Autodesk Inventor part; units mm, degrees
ref_plane "Work Plane1" through (-106.5, -37, 0) normal (1, 0, 0) x (0, 1, 0)
ref_plane "Work Plane2" through (-183, -37, 0) normal (1, 0, 0) x (0, 1, 0)
ref_plane "Work Plane3" through (-106.5, -37, -17.5) normal (0, -1, 0) x (1, 0, 0)
sketch "Sketch1" plane through (0, 0, 0) normal (0, 0, 1) x (1, 0, 0)
  line L0 (-183, -19.5) -> (-106.5, -19.5)
  line L1 (-106.5, -19.5) -> (-106.5, -54.5)
  line L2 (-106.5, -54.5) -> (-183, -54.5)
  line L3 (-183, -54.5) -> (-183, -19.5)
  line L4 (-194, -37) -> (-96, -37) construction
  line L5 (-183, -22) -> (-157.5, -22)
  line L6 (-157.5, -22) -> (-157.5, -37)
  line L7 (-157.5, -24.5) -> (-116.5, -24.5)
  line L8 (-116.5, -37) -> (-116.5, -22)
  line L9 (-116.5, -22) -> (-106.5, -22)
  line L10 (-183, -52) -> (-157.5, -52) construction
  line L11 (-157.5, -52) -> (-157.5, -37) construction
  line L12 (-157.5, -49.5) -> (-116.5, -49.5) construction
  line L13 (-116.5, -37) -> (-116.5, -52) construction
  line L14 (-116.5, -52) -> (-106.5, -52) construction
  line L15 (-183, -37) -> (-106.5, -37)
  point P0 (0, 0)
  dimension "d0" = 76.5
  dimension "d1" = 35
  dimension "d2" = 30
  dimension "d3" = 25.5
  dimension "d4" = 10
  dimension "d5" = 25
  dimension "d6" = 30
sketch "Sketch3" plane through (0, 0, 0) normal (1, 0, 0) x (0, 1, 0)
  point P0 (0, 0)
ref_plane "Work Plane1" through (-106.5, -37, 0) normal (1, 0, 0) x (0, 1, 0)
sketch "Sketch4" plane through (-106.5, -37, 0) normal (1, 0, 0) x (0, 1, 0)
  point P0 (37, 0)
sketch "Sketch5" plane through (-106.5, -37, 0) normal (1, 0, 0) x (0, 1, 0)
  line L0 (-17.5, 17.5) -> (17.5, 17.5)
  line L1 (17.5, 17.5) -> (17.5, -17.5)
  line L2 (17.5, -17.5) -> (-17.5, -17.5)
  line L3 (-17.5, -17.5) -> (-17.5, 17.5)
  line L4 (-17.5, 17.5) -> (17.5, -17.5) construction
  line L5 (17.5, 17.5) -> (-17.5, -17.5) construction
  point P0 (37, 0)
  point P1 (0, 0)
  dimension "d10" = 35
  dimension "d11" = 35
ref_plane "Work Plane2" through (-183, -37, 0) normal (1, 0, 0) x (0, 1, 0)
extrude "Extrusion1" add sketch "Sketch5" against normal up to surface (76.5 mm away)
revolve "Revolution2" cut sketch "Sketch1" angle 360 about axis through (-194, -37, 0) along (1, 0, 0) contours L5 L6 L15 L3 | L1 L15 L8 L9 | L6 L7 L8 L15
sketch "Sketch7" plane through (-106.5, -37, 0) normal (1, 0, 0) x (0, 0, -1)
  circle A0 centre (0, 0) radius 19.09
  line L0 (-17.5, -17.5) -> (17.5, -17.5)
  line L1 (-17.5, 17.5) -> (-17.5, -17.5)
  line L2 (17.5, -17.5) -> (-17.5, 17.5) construction
  circle A1 centre (13.4987, -13.4987) radius 1.5
  circle A2 centre (13.4987, 13.4987) radius 1.5
  circle A3 centre (-13.4987, 13.4987) radius 1.5
  circle A4 centre (-13.4987, -13.4987) radius 1.5
  point P0 (0, 37)
  dimension "d21" = 38.18
  dimension "d22" = 3
  dimension "d25" = 360
hole "Hole1" at (-106.5, -23.5013, -13.4987) at (-106.5, -23.5013, 13.4987) at (-106.5, -50.4987, 13.4987) at (-106.5, -50.4987, -13.4987) direction (-1, 0, 0) diameter 2.8 depth 7 tip angle 118 counterbore diameter 3 counterbore depth 5
sketch "Sketch8" plane through (-183, -54.5, -17.5) normal (-1, 0, 0) x (0, 0, 1)
  line L0 (17.5, -7) -> (17.5, 46)
  circle A0 centre (2.5, 30) radius 1.25
  line L1 (0, 35) -> (0, 0)
  line L2 (35, 35) -> (0, 35)
  circle A1 centre (32.5, 30) radius 1.25
  circle A2 centre (17.5, 17.5) radius 15
  circle A3 centre (17.5, 17.5) radius 15
  line L3 (5.3, 6.5) -> (5.3, 35)
  line L4 (0, 35) -> (35, 35)
  arc A4 (5.3, 6.5) -> (6.3, 5.5) centre (6.3, 6.5) ccw
  line L5 (17.5, 5.5) -> (6.3, 5.5)
  line L6 (29.7, 6.5) -> (29.7, 35)
  arc A5 (28.7, 5.5) -> (29.7, 6.5) centre (28.7, 6.5) ccw
  line L7 (17.5, 5.5) -> (28.7, 5.5)
  point P0 (17.5, 54.5)
  point P1 (17.5, 5.5)
  point P2 (5.3, 35)
  dimension "d34" = 2.5
  dimension "d35" = 2.5
  dimension "d36" = 5
  dimension "d38" = 1
  dimension "d39" = 29.5
  dimension "d40" = 24.4
extrude "Extrusion2" cut sketch "Sketch8" against normal blind 2.75 contours L5 A2 L3 L0 | L0 A2 L6 L7 | L5 A4 L3 A2 | A2 L6 A5 L7 | A2 L3 L2 L0 | L0 L2 L6 A2
hole "Hole2" at (-183, -24.5, -15) at (-183, -24.5, 15) direction (1, 0, 0) diameter 2 depth 5 tip angle 118 counterbore diameter 2.5 counterbore depth 4
ref_plane "Work Plane3" through (-106.5, -37, -17.5) normal (0, -1, 0) x (1, 0, 0)
sketch "Sketch9" plane through (-106.5, -37, -17.5) normal (0, -1, 0) x (1, 0, 0)
  point P0 (106.5, 17.5)
sketch "Sketch11" plane through (-106.5, -19.5, 17.5) normal (0, 1, 0) x (1, 0, 0)
  line L0 (-73.75, 5.3) -> (-76.5, 5.3)
  line L1 (-76.5, 0) -> (-76.5, 5.3)
  line L2 (0, 0) -> (-76.5, 0)
  line L3 (0, 35) -> (0, 0)
  line L4 (0, 35) -> (-76.5, 35)
  line L5 (-76.5, 29.7) -> (-76.5, 35)
  line L6 (-76.5, 29.7) -> (-73.75, 29.7)
  line L7 (-73.75, 29.7) -> (-73.75, 5.3)
  line L8 (28.2317, 17.5) -> (-103.7683, 17.5) construction
  circle A0 centre (-30, 17.5) radius 1.5
  circle A1 centre (-50, 17.5) radius 2.5
  point P0 (106.5, 17.5)
  point P1 (0, 17.5)
  dimension "d54" = 3
  dimension "d55" = 5
  dimension "d56" = 30
  dimension "d57" = 50
extrude "Extrusion3" cut sketch "Sketch11" against normal up to surface (35 mm away) contours A0
extrude "Extrusion4" cut sketch "Sketch11" against normal up to surface contours A1
sketch "Sketch12" plane through (-106.5, -54.5, -17.5) normal (0, 0, -1) x (-1, 0, 0)
  line L0 (76.5, 35) -> (76.5, 0)
  line L1 (0, 35) -> (76.5, 35)
  line L2 (0, 0) -> (0, 35)
  line L3 (0, 0) -> (76.5, 0)
  line L4 (-16, 17.5) -> (90, 17.5)
  circle A0 centre (15, 5) radius 1.5
  circle A1 centre (45, 5) radius 1.5
  circle A2 centre (15, 30) radius 1.5
  circle A3 centre (45, 30) radius 1.5
  point P0 (-106.5, 54.5)
  point P1 (0, 17.5)
  dimension "d62" = 3
  dimension "d63" = 15
  dimension "d64" = 5
  dimension "d67" = 30
hole "Hole3" at (-121.5, -24.5, -17.5) at (-151.5, -24.5, -17.5) at (-151.5, -49.5, -17.5) at (-121.5, -49.5, -17.5) direction (0, 0, 1) diameter 2.8 depth 7 tip angle 118 counterbore diameter 3 counterbore depth 5
ref_plane "Work Plane4" through (-106.5, -54.5, 0) normal (0, 0, -1) x (-1, 0, 0)
mirror "Mirror2" about plane through (-106.5, -54.5, 0) normal (0, 0, -1) of "Hole3"
chamfer "Chamfer3" distance 0.5 angle 45 4 edges at (-151.5, -51, -17.5) (-151.5, -26, -17.5) (-121.5, -51, -17.5) (-121.5, -26, -17.5) measured on face at (-172.9115, -40.8826, -17.5)
chamfer "Chamfer4" distance 0.5 angle 45 4 edges at (-151.5, -26, 17.5) (-151.5, -51, 17.5) (-121.5, -26, 17.5) (-121.5, -51, 17.5) measured on face at (-172.9115, -33.1174, 17.5)
chamfer "Chamfer5" distance 0.5 angle 45 4 edges at (-106.5, -50.4987, -11.9987) (-106.5, -23.5013, -11.9987) (-106.5, -50.4987, 14.9987) (-106.5, -23.5013, 14.9987) measured on face at (-106.5, -37.6027, 16.6302)
chamfer "Chamfer6" distance 0.2 angle 45 1 edges at (-159, -19.5, 0) measured on face at (-148.5662, -19.5, -12.4939)
equation "\"d27\" = m3"
equation "\"d72\" = m3"
equation "\"m3\" = 2.8"
equation "\"m4\" = 3.8"
properties part number "АНЦП.014.00.00.003" material "PET Plastic"
CAD build for the part. Positions are in the model's coordinates, mm. A direction names the side the tool comes from. Coordinates: 2 decimals unless noted, no trailing zeros. Order: outer loops, then holes, each group sorted by start corner. A loop starts at its lowest first (then second) coordinate and runs counter-clockwise, first axis right, second up. Notation, with made-up numbers: (22.25, -27.75) -> (66.25, -27.75) arc R19 cw to (66.25, -8.75) -> close; hole circle Ø10 at (19.25, 62). An arc over 180 degrees is marked (long way). Answer in a Markdown table with one row per item.
1) Band-saw the part on C-C (z = -6). List the corners of the cut face in (x, y).
Check values:
| item | result |
|---|---|
| outline | (-183, -54.5) -> (-106.5, -54.5) -> (-106.5, -50.75) -> (-116.5, -50.75) -> (-116.5, -47.97) -> (-157.5, -47.97) -> (-157.5, -50.75) -> (-183, -50.75) -> close; (-180.25, -23.25) -> (-157.5, -23.25) -> (-157.5, -26.03) -> (-116.5, -26.03) -> (-116.5, -23.25) -> (-106.5, -23.25) -> (-106.5, -19.5) -> (-180.25, -19.5) -> close |
2) Band-saw the part on B-B (x = -136.5). List the corners of the cut face in (y, z), and give its area (3 significant figures).
Check values:
| item | result |
|---|---|
| outline | (-54.5, -17.5) -> (-19.5, -17.5) -> (-19.5, -1.5) -> (-24.59, -1.5) arc R12.5 cw to (-49.41, -1.5) -> (-54.5, -1.5) -> close; (-54.5, 1.5) -> (-49.41, 1.5) arc R12.5 cw to (-24.59, 1.5) -> (-19.5, 1.5) -> (-19.5, 17.5) -> (-54.5, 17.5) -> close |
| area | 704 mm2 |
3) Flat gauge pins, fed straight in: P1, Ø1.5, axis at y = -24.5, z = -15, coming from the -X side; P2, Ø2.5, axis at x = -151.5, y = -24.5, coming from the +Z side; P3, Ø0.9, axis at x = -121.5, y = -49.5, coming from the +Z side. Where does each tip first touch, or does it go through?
Check values:
| item | result |
|---|---|
| P1 | x = -177.85 |
| P2 | z = 10.41 |
| P3 | z = 9.93 |
4) Band-saw the part on D-D (x = -160). List the corners of the cut face in (y, z), and give its area (3 significant figures).
Check values:
| item | result |
|---|---|
| outline | (-54.5, -17.5) -> (-19.5, -17.5) -> (-19.5, 17.5) -> (-54.5, 17.5) -> close; hole circle Ø30 at (-37, 0) |
| area | 518 mm2 |
5) Which spindle directions (+Z, -Z, +X, -X, +Y, -Y) get a long thin tool onto all of the face, cutting with end or side? Do faces 1 (the face through (-122.89, -24.68, -11.49)), 2 (the face through (-112.51, -24.45, -12.47)), 3 (the face through (-182, -49, 10)), 4 (the face through (-150.32, -48.75, 11.49)). Say none if no direction does.
Check values:
| item | result |
|---|---|
| face 1 | -Z |
| face 2 | +X |
| face 3 | -X, +Y |
| face 4 | +Z |
6) Band-saw the part on A-A (y = -37). List the corners of the cut face in (x, z), and give its area (4 significant figures).
Check values:
| item | result |
|---|---|
| outline | (-183, -17.5) -> (-106.5, -17.5) -> (-106.5, -15) -> (-116.5, -15) -> (-116.5, -12.5) -> (-157.5, -12.5) -> (-157.5, -15) -> (-183, -15) -> close; (-183, 15) -> (-157.5, 15) -> (-157.5, 12.5) -> (-116.5, 12.5) -> (-116.5, 15) -> (-106.5, 15) -> (-106.5, 17.5) -> (-183, 17.5) -> close |
| area | 587.5 mm2 |
7) Mould opens along Y. For faces 5 (the face through (-144, -37, -17.5)), 6 (the face through (-178.49, -23.61, -14.54)), 7 (the face through (-182, -49, -10)) say: pulls with the +Y half, pulls with the -Y half, needs draft (parallel to the pull), parting line crosses it, or undercut.
Check values:
| item | result |
|---|---|
| face 5 | needs draft |
| face 6 | undercut |
| face 7 | pulls with the +Y half |
8) Drill centre lines: line 1 (Y direction, x = -151.5, z = 14.8); line 2 (Y direction, x = -121, z = -14); line 3 (X direction, y = -21.2, z = 0). Where is each one in solid material? Low to high.
Check values:
| item | result |
|---|---|
| line 1 | -54.5 to -51, -48 to -26, -23 to -19.5 |
| line 2 | -54.5 to -50.91, -48.09 to -25.91, -23.09 to -19.5 |
| line 3 | -180.25 to -159, -154 to -138, -135 to -106.5 |
